Autodesk Inventor part; units mm, degrees
ref_plane "YZ Plane" through (0, 0, 0) normal (1, 0, 0) x (0, 1, 0)
ref_plane "XZ Plane" through (0, 0, 0) normal (0, 1, 0) x (-1, 0, 0)
ref_plane "XY Plane" through (0, 0, 0) normal (0, 0, 1) x (1, 0, 0)
sketch "Sketch1" plane through (0, 0, 0) normal (0, 0, 1) x (1, 0, 0)
  line L0 (-15, 19) -> (-15, -19)
  arc A0 (-10, 24) -> (-15, 19) centre (-10, 19) ccw
  line L1 (10, 24) -> (-10, 24)
  arc A1 (15, 19) -> (10, 24) centre (10, 19) ccw
  line L2 (15, -19) -> (15, 19)
  arc A2 (10, -24) -> (15, -19) centre (10, -19) ccw
  line L3 (-10, -24) -> (10, -24)
  arc A3 (-15, -19) -> (-10, -24) centre (-10, -19) ccw
  point P0 (0, 0)
extrude "Extrusion1" add sketch "Sketch1" along normal blind 10
sketch "Sketch2" plane through (0, 0, 0) normal (0, 0, -1) x (-1, 0, 0)
  circle A0 centre (-10, 19) radius 1.6
  circle A1 centre (-10, -19) radius 1.6
  arc A2 (10, -24) -> (15, -19) centre (10, -19) ccw
  line L0 (15, 19) -> (15, -19)
  arc A3 (15, 19) -> (10, 24) centre (10, 19) ccw
  line L1 (-10, 24) -> (10, 24)
  arc A4 (-10, 24) -> (-15, 19) centre (-10, 19) ccw
  line L2 (-15, -19) -> (-15, 19)
  arc A5 (-15, -19) -> (-10, -24) centre (-10, -19) ccw
  line L3 (10, -24) -> (-10, -24)
  circle A6 centre (10, -19) radius 1.6
  circle A7 centre (10, 19) radius 1.6
hole "Hole1" at (10, 19, 0) at (10, -19, 0) at (-10, -19, 0) at (-10, 19, 0) direction (0, 0, 1) diameter 2.459 depth 8 tip angle 118
sketch "Sketch3" plane through (0, 0, 0) normal (0, 0, -1) x (-1, 0, 0)
  circle A0 centre (10, 19) radius 1.2295 construction
  circle A1 centre (10, -19) radius 1.2295 construction
  circle A2 centre (-10, -19) radius 1.2295 construction
  circle A3 centre (-10, 19) radius 1.2295 construction
  arc A4 (10, -24) -> (15, -19) centre (10, -19) ccw
  line L0 (15, 19) -> (15, -19)
  arc A5 (15, 19) -> (10, 24) centre (10, 19) ccw
  line L1 (-10, 24) -> (10, 24)
  arc A6 (-10, 24) -> (-15, 19) centre (-10, 19) ccw
  line L2 (-15, -19) -> (-15, 19)
  arc A7 (-15, -19) -> (-10, -24) centre (-10, -19) ccw
  line L3 (10, -24) -> (-10, -24)
  arc A8 (15, 19) -> (10, 24) centre (10, 19) ccw
  line L4 (-10, 24) -> (10, 24)
  arc A9 (-10, 24) -> (-15, 19) centre (-10, 19) ccw
  line L5 (-15, -19) -> (-15, 19)
  arc A10 (-15, -19) -> (-10, -24) centre (-10, -19) ccw
  line L6 (10, -24) -> (-10, -24)
  arc A11 (10, -24) -> (15, -19) centre (10, -19) ccw
  line L7 (15, 19) -> (15, -19)
  circle A12 centre (11.6971, -20.6971) radius 0.25 construction
  circle A13 centre (12.4, -19) radius 0.25 construction
  circle A14 centre (10, -21.4) radius 0.25 construction
  circle A15 centre (10, -19) radius 1.6 construction
  circle A16 centre (11.6971, -17.3029) radius 0.25 construction
  circle A17 centre (10, -16.6) radius 0.25 construction
  circle A18 centre (8.3029, -20.6971) radius 0.25 construction
  circle A19 centre (7.6, -19) radius 0.25 construction
  circle A20 centre (8.3029, -17.3029) radius 0.25 construction
  circle A21 centre (2.62, -11.54) radius 0.5 construction
  circle A22 centre (0.08, -11.54) radius 0.5 construction
  circle A23 centre (11.3, -10.4) radius 0.4953 construction
  circle A24 centre (12.316, -5.32) radius 0.4953 construction
  circle A25 centre (10.284, -5.32) radius 0.4953 construction
  circle A26 centre (2.62, -9) radius 0.5 construction
  circle A27 centre (0.08, -9) radius 0.5 construction
  circle A28 centre (-2.46, -11.54) radius 0.5 construction
  circle A29 centre (-8.3029, -20.6971) radius 0.25 construction
  circle A30 centre (-7.6, -19) radius 0.25 construction
  circle A31 centre (-10, -21.4) radius 0.25 construction
  circle A32 centre (-10, -19) radius 1.6 construction
  circle A33 centre (-8.3029, -17.3029) radius 0.25 construction
  circle A34 centre (-10, -16.6) radius 0.25 construction
  circle A35 centre (-11.6971, -20.6971) radius 0.25 construction
  circle A36 centre (-12.4, -19) radius 0.25 construction
  circle A37 centre (-11.6971, -17.3029) radius 0.25 construction
  circle A38 centre (-2.46, -9) radius 0.5 construction
  circle A39 centre (-13.3, -3.2) radius 0.45 construction
  circle A40 centre (-13.3, -0.2) radius 0.45 construction
  circle A41 centre (10.7, 8.9) radius 0.1 construction
  circle A42 centre (9.85, 8.9) radius 0.1 construction
  circle A43 centre (10.7, 9.7) radius 0.1 construction
  circle A44 centre (9.85, 9.7) radius 0.1 construction
  circle A45 centre (9, 8.9) radius 0.1 construction
  circle A46 centre (9, 9.7) radius 0.1 construction
  circle A47 centre (11.6971, 17.3029) radius 0.25 construction
  circle A48 centre (12.4, 19) radius 0.25 construction
  circle A49 centre (10, 16.6) radius 0.25 construction
  circle A50 centre (10, 19) radius 1.6 construction
  circle A51 centre (11.6971, 20.6971) radius 0.25 construction
  circle A52 centre (10, 21.4) radius 0.25 construction
  circle A53 centre (8.3029, 17.3029) radius 0.25 construction
  circle A54 centre (7.6, 19) radius 0.25 construction
  circle A55 centre (8.3029, 20.6971) radius 0.25 construction
  arc A56 (4.02, 16.62) -> (4.62, 16.62) centre (4.32, 16.62) ccw construction
  line L8 (4.02, 17.72) -> (4.02, 16.62) construction
  arc A57 (4.62, 17.72) -> (4.02, 17.72) centre (4.32, 17.72) ccw construction
  line L9 (4.62, 16.62) -> (4.62, 17.72) construction
  circle A58 centre (2.89, 17.7) radius 0.325 construction
  arc A59 (4.02, 21.05) -> (4.62, 21.05) centre (4.32, 21.05) ccw construction
  line L10 (4.02, 21.65) -> (4.02, 21.05) construction
  arc A60 (4.62, 21.65) -> (4.02, 21.65) centre (4.32, 21.65) ccw construction
  line L11 (4.62, 21.05) -> (4.62, 21.65) construction
  circle A61 centre (-2.89, 17.7) radius 0.325 construction
  arc A62 (-4.62, 16.62) -> (-4.02, 16.62) centre (-4.32, 16.62) ccw construction
  line L12 (-4.62, 17.72) -> (-4.62, 16.62) construction
  arc A63 (-4.02, 17.72) -> (-4.62, 17.72) centre (-4.32, 17.72) ccw construction
  line L13 (-4.02, 16.62) -> (-4.02, 17.72) construction
  arc A64 (-4.62, 21.05) -> (-4.02, 21.05) centre (-4.32, 21.05) ccw construction
  line L14 (-4.62, 21.65) -> (-4.62, 21.05) construction
  arc A65 (-4.02, 21.65) -> (-4.62, 21.65) centre (-4.32, 21.65) ccw construction
  line L15 (-4.02, 21.05) -> (-4.02, 21.65) construction
  circle A66 centre (-8.3029, 17.3029) radius 0.25 construction
  circle A67 centre (-7.6, 19) radius 0.25 construction
  circle A68 centre (-10, 16.6) radius 0.25 construction
  circle A69 centre (-10, 19) radius 1.6 construction
  circle A70 centre (-8.3029, 20.6971) radius 0.25 construction
  circle A71 centre (-10, 21.4) radius 0.25 construction
  circle A72 centre (-11.6971, 17.3029) radius 0.25 construction
  circle A73 centre (-12.4, 19) radius 0.25 construction
  circle A74 centre (-11.6971, 20.6971) radius 0.25 construction
  line L16 (11.3, -10.4) -> (11.3, -5.32) construction
  line L17 (13.8, -10.4) -> (13.8, -5.32)
  line L18 (8.8, -5.32) -> (8.8, -10.4)
  arc A75 (8.8, -10.4) -> (13.8, -10.4) centre (11.3, -10.4) ccw
  arc A76 (13.8, -5.32) -> (8.8, -5.32) centre (11.3, -5.32) ccw
  line L19 (11.3, -5.32) -> (12.316, -5.32) construction
  line L20 (-4.32, 17.72) -> (4.32, 17.72) construction
  line L21 (4.32, 21.05) -> (-4.32, 21.05) construction
  line L22 (0, 17.72) -> (0, 21.05) construction
  line L23 (-4, 19.385) -> (4, 19.385) construction
  line L24 (-4, 15.885) -> (4, 15.885)
  line L25 (4, 22.885) -> (-4, 22.885)
  arc A77 (-4, 22.885) -> (-4, 15.885) centre (-4, 19.385) ccw
  arc A78 (4, 15.885) -> (4, 22.885) centre (4, 19.385) ccw
  line L26 (-2.46, -11.54) -> (2.62, -9) construction
  line L27 (2.62, -11.54) -> (-2.46, -9) construction
  line L28 (-2.92, -10.27) -> (3.08, -10.27) construction
  line L29 (-2.92, -14.27) -> (3.08, -14.27)
  line L30 (3.08, -6.27) -> (-2.92, -6.27)
  arc A79 (-2.92, -6.27) -> (-2.92, -14.27) centre (-2.92, -10.27) ccw
  arc A80 (3.08, -14.27) -> (3.08, -6.27) centre (3.08, -10.27) ccw
  point P0 (0, 0)
  point P1 (11.3, -7.86)
  point P2 (0, 19.385)
  point P3 (0.08, -10.27)
  dimension "d10" = 5
  dimension "d16" = 4
  dimension "d17" = 7
  dimension "d18" = 3
  dimension "d19" = 8
extrude "Extrusion2" cut sketch "Sketch3" against normal blind 5 contours A75 L18 A76 L17 | A77 L25 A78 L24 | A79 L30 A80 L29
properties part number "Backplate" material "Aluminum 6061"
Geometry check sheet. Reference: the model listing, model coordinates, mm. A direction names the side the tool comes from. Coordinates: 2 decimals unless noted, no trailing zeros. Order: outer loops, then holes, each group sorted by start corner. A loop starts at its lowest first (then second) coordinate and runs counter-clockwise, first axis right, second up.
Q1. Thickness scan on probe 1 along Y at (x, z) = (10, 3.5); probe 2 along Y at (x, z) = (-0.75, 1) (3 decimals); probe 3 along X at (y, z) = (-19, 2.5). Record the ranges inside material, lowest first.
Reply:
probe 1: y = -24 to -20.23, -17.77 to 17.77, 20.23 to 24
probe 2: y = -24 to -14.27, -6.27 to 15.885, 22.885 to 24
probe 3: x = -15 to -11.23, -8.77 to 8.77, 11.23 to 15
Q2. Sectioned sample at A-A on z = 7. Record the cut outline in (x, y), and give its area (3 significant figures).
Reply:
outline: (-15, -19) arc R5 ccw to (-10, -24) - (10, -24) arc R5 ccw to (15, -19) - (15, 19) arc R5 ccw to (10, 24) - (-10, 24) arc R5 ccw to (-15, 19) - close; hole circle Ø2.46 at (-10, -19); hole circle Ø2.46 at (-10, 19); hole circle Ø2.46 at (10, -19); hole circle Ø2.46 at (10, 19)
area: 1,400 mm2
Q3. Tool access check on faces 5 (the face through (15, 0, 5)), 6 (the face through (0, -10, 5)). Record the directions out of +Z, -Z, +X, -X, +Y, -Y that give a thin tool (end or side, any length) a straight path to the whole face; none if there is none.
Reply:
face 5: +Z, -Z, +X, +Y, -Y
face 6: -Z
Q4. Depth check by flat-ended pin: pin 1 Ø2.5 at (x, y) = (-11.5, -9.5) entering from -Z. Enter the tip coordinate at first touch or a pass-through.
Reply:
pin 1: stops at z = 5
Q5. Draft check along X on faces 1 (the face through (-9.936, 19.204, 8.61)), 2 (the face through (0, 0, 0)), 3 (the face through (10.471, 20.136, 4.056)), 4 (the face through (13, 23, 5)). Enter one of: released by +X, released by -X, zero draft, split by the parting line, or undercut.
Reply:
face 1: undercut
face 2: zero draft
face 3: undercut
face 4: released by +X
Q6. Sectioned sample at B-B on x = 5. Record the cut outline in (y, z).
Reply:
outline: (-24, 0) - (-13.69, 0) - (-13.69, 5) - (-6.85, 5) - (-6.85, 0) - (16.03, 0) - (16.03, 5) - (22.74, 5) - (22.74, 0) - (24, 0) - (24, 10) - (-24, 10) - close
Q7. Sectioned sample at C-C on y = -7. Record the cut outline in (x, z), and give its area (3 significant figures).
Reply:
outline: (-15, 0) - (-13.8, 0) - (-13.8, 5) - (-8.8, 5) - (-8.8, 0) - (-5.38, 0) - (-5.38, 5) - (5.22, 5) - (5.22, 0) - (15, 0) - (15, 10) - (-15, 10) - close
area: 222 mm2
